Work out the finished part from the listing and answer in its coordinate system (mm). A direction names the side the tool comes from. Give positions to 0.01 mm unless a question says otherwise; leave off trailing zeros. Loops run counter-clockwise (first coordinate to the right, second up) from the corner with the lowest first, then second, coordinate; pieces in that order, holes last. Notation, with made-up numbers: M 87.5,75.25 L 91.5,75.25 A23 ccw 91.5,91.25 Z; hole C 15.25,15 d7. An arc over 180 degrees is marked long. Answer as a JSON object with one key per item and string values. Group by question number.
Autodesk Inventor part; units mm, degrees
ref_plane "YZ Plane" through (0, 0, 0) normal (1, 0, 0) x (0, 1, 0)
ref_plane "XZ Plane" through (0, 0, 0) normal (0, 1, 0) x (-1, 0, 0)
ref_plane "XY Plane" through (0, 0, 0) normal (0, 0, 1) x (1, 0, 0)
sketch "Esboço1" plane through (0, 0, 0) normal (0, 0, 1) x (1, 0, 0)
  line L0 (3.6169, 102.1463) -> (3.6169, -101.8537)
  line L1 (-13.8831, -106.8537) -> (-13.8831, 106.8093)
  line L2 (-13.8831, -106.8537) -> (-4.3831, -106.8537)
  line L3 (-13.8831, 106.8093) -> (-4.3831, 106.8093)
  circle A0 centre (-9.1331, -96.8537) radius 1.621
  circle A1 centre (-9.1331, -0.0222) radius 1.621
  circle A2 centre (-9.1331, 96.8093) radius 1.621
  line L4 (-13.8831, -106.8537) -> (13.6169, -106.8537)
  line L5 (13.6169, -106.8537) -> (13.6169, 106.8093)
  line L6 (13.6169, 106.8093) -> (-13.8831, 106.8093)
  line L7 (-13.8831, 106.8093) -> (-13.8831, -106.8537)
  point P0 (0, 0)
  point P1 (-13.8831, -10.6907)
  dimension "d0" = 0
  dimension "d1" = 10
extrude "Extrusão1" add sketch "Esboço1" along normal blind 9.5
sketch "Esboço2" plane through (0, 0, 0) normal (0, 0, -1) x (-1, 0, 0)
  line L0 (-13.6169, 106.8093) -> (13.8831, 106.8093)
  line L1 (13.8831, -106.8537) -> (-13.6169, -106.8537)
  line L2 (-13.6169, 106.8093) -> (-4.1169, 106.8093)
  line L3 (-4.1169, 106.8093) -> (-4.1169, -106.8537)
  line L4 (-4.1169, -106.8537) -> (-13.6169, -106.8537)
  line L5 (-13.6169, -106.8537) -> (-13.6169, 106.8093)
  point P0 (0, 0)
  dimension "d4" = 9.5
extrude "Extrusão2" add sketch "Esboço2" along normal blind 15
sketch "Esboço3" plane through (0, 0, 9.5) normal (0, 0, 1) x (1, 0, 0)
  circle A0 centre (-9.1331, -96.8537) radius 1.621
  circle A1 centre (-9.1331, -0.0222) radius 1.621
  circle A2 centre (-9.1331, 96.8093) radius 1.621
  point P0 (0, 0)
hole "Furo1" at (-9.1331, -96.8537, 9.5) at (-9.1331, -0.0222, 9.5) at (-9.1331, 96.8093, 9.5) direction (0, 0, -1) diameter 4.5 end through all
properties part number "Guia lateral do top" material "Alumínio 6061"
Item 1: Find the intervals of material crossed by probe 1 along Z at (x, y) = (-1.75, -71); probe 2 along X at (y, z) = (-57, -8), in increasing order. Write a range as [from, to].
Item 2: Given pin 1 Ø2.5 at (x, y) = (-9.13, 96.81) entering from -Z; pin 2 Ø14.5 at (x, y) = (-8.5, 18.5) entering from -Z; pin 3 Ø1 at (y, z) = (-59, -8.5) entering from -X, each flat-ended and moving along its own axis, determine where each tip first touches the part or whether it passes through.
Item 3: For a pull along Y with two mould halves and no side action, classify faces 3 (the flat face through (4.117, 1, -7)), 4 (the flat face through (3, -106.854, 3)), 5 (the cylindrical face through (-9.232, 99.057, 4.684)) as pulls with the +Y half, pulls with the -Y half, needs draft (parallel to the pull), parting line crosses it, or undercut.
Item 4: A cutting plane is placed at B-B (z = -2.5). Determine the outline of the cut face in (x, y).
Item 5: A tool of negligible diameter and unlimited length cuts with its end or side. For faces 1 (the flat face through (-5, 1, 0)), 2 (the flat face through (9, 1, -15)), from which of +Z, -Z, +X, -X, +Y, -Y can it reach the whole face along a straight path? Write none if from no direction.
Item 6: A cutting plane is placed at A-A (y = -73). Determine the outline of the cut face in (x, z).
Item 7: A cutting plane is placed at C-C (x = 1.25). Determine the outline of the cut face in (y, z).
The answers:
{
 "1": {"probe 1": "z = [0, 9.5]", "probe 2": "x = [4.12, 13.62]"},
 "2": {"pin 1": "passes through", "pin 2": "stops at z = 0", "pin 3": "stops at x = 4.12"},
 "3": {"face 3": "needs draft", "face 4": "pulls with the -Y half", "face 5": "undercut"},
 "4": {"outline": "M 4.12,-106.85 L 13.62,-106.85 L 13.62,106.81 L 4.12,106.81 Z"},
 "5": {"face 1": "-Z, -X, +Y, -Y", "face 2": "-Z, +X, -X, +Y, -Y"},
 "6": {"outline": "M -13.88,0 L 4.12,0 L 4.12,-15 L 13.62,-15 L 13.62,9.5 L -13.88,9.5 Z"},
 "7": {"outline": "M -106.85,0 L 106.81,0 L 106.81,9.5 L -106.85,9.5 Z"}
}
